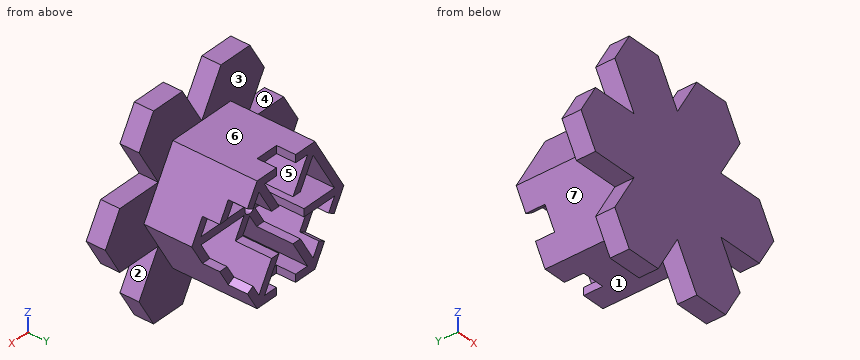
from build123d import *

# Parameters (mm, degrees)
SALIENTE_EXTRUIR1_DEPTH = 10
SALIENTE_EXTRUIR2_DEPTH = 170
CORTAR_EXTRUIR1_DEPTH   = 4
MATRIZC1_COUNT          = 5
MATRIZC1_ANGLE          = 240
CROQUIS4_W              = 24
CROQUIS4_H              = 12
SALIENTE_EXTRUIR3_DEPTH = 36
CROQUIS5_W              = 24
CROQUIS5_H              = 9
CORTAR_EXTRUIR2_DEPTH   = 24
CHAFL_N1_SIZE2          = 36
CHAFL_N1_SIZE           = 98.9091871
CORTAR_EXTRUIR3_DEPTH   = 24
CROQUIS7_W              = 30
CROQUIS7_H              = 18
CROQUIS7_R              = 3
SALIENTE_EXTRUIR4_DEPTH = 3
CROQUIS8_W              = 150
CROQUIS8_H              = 150
CORTAR_EXTRUIR4_DEPTH   = 130
CROQUIS9_W              = 64.5
CROQUIS9_H              = 23
CORTAR_EXTRUIR5_DEPTH   = 19
CROQUIS10_R             = 3
CORTAR_EXTRUIR6_DEPTH   = 8


with BuildPart() as part:
    # Croquis1 → Saliente-Extruir1 (new body)
    with BuildSketch(Plane(origin=(0, 0, 0), x_dir=(1, 0, 0), z_dir=(0, 1, 0))):
        Polygon((-12, 51.961524227), (-30, 51.961524227), (-39, 36.373066959), (-27, 15.588457268), (-51, 15.588457268), (-60, 0), (-51, -15.588457268), (-27, -15.588457268), (-39, -36.373066959), (-30, -51.961524227), (-12, -51.961524227), (0, -31.176914536), (12, -51.961524227), (30, -51.961524227), (39, -36.373066959), (27, -15.588457268), (51, -15.588457268), (60, 0), (51, 15.588457268), (27, 15.588457268), (39, 36.373066959), (30, 51.961524227), (12, 51.961524227), (0, 31.176914536), align=None)
    extrude(amount=SALIENTE_EXTRUIR1_DEPTH)

    # Croquis2 → Saliente-Extruir2 (add)
    # profile 1 of 2: a face of its own
    with BuildSketch(Plane(origin=(0, 10, 0), x_dir=(1, 0, 0), z_dir=(0, 1, 0))):
        Polygon((36, 0), (18, 31.176914536), (-18, 31.176914536), (-36, 0), (-18, -31.176914536), (18, -31.176914536), align=None)
        Polygon((15.690598923, 27.176914536), (-15.690598923, 27.176914536), (-31.381197846, 0), (-15.690598923, -27.176914536), (15.690598923, -27.176914536), (31.381197846, 0), align=None, mode=Mode.SUBTRACT)
    # profile 2 of 2: a face of its own
    with BuildSketch(Plane(origin=(0, 10, 0), x_dir=(1, 0, 0), z_dir=(0, 1, 0))):
        Polygon((-13.381197846, 27.176914536), (-15.690598923, 27.176914536), (-16.845299462, 25.176914536), (-3.464101615, 2), (-30.226497308, 2), (-31.381197846, 0), (-30.226497308, -2), (-3.464101615, -2), (-16.845299462, -25.176914536), (-15.690598923, -27.176914536), (-13.381197846, -27.176914536), (0, -4), (13.381197846, -27.176914536), (15.690598923, -27.176914536), (16.845299462, -25.176914536), (3.464101615, -2), (30.226497308, -2), (31.381197846, 0), (30.226497308, 2), (3.464101615, 2), (16.845299462, 25.176914536), (15.690598923, 27.176914536), (13.381197846, 27.176914536), (0, 4), align=None)
    extrude(amount=SALIENTE_EXTRUIR2_DEPTH)

    # Croquis3 → Cortar-Extruir1 (cut)
    with BuildSketch(Plane.XY.offset(31.176914536)):
        Polygon((-14, 172), (-2, 172), (6, 164), (6, 44), (-6, 44), (-6, 159.029437252), (-6.970562748, 160), (-14, 160), align=None)
    cortar_extruir1 = extrude(amount=-CORTAR_EXTRUIR1_DEPTH, mode=Mode.SUBTRACT)

    # MatrizC1: Cortar-Extruir1 ×5 about axis
    matrizc1_axis = Axis((0, 0, 0), (0, 1, 0))
    for i in range(1, MATRIZC1_COUNT):
        add(cortar_extruir1.rotate(matrizc1_axis, i * MATRIZC1_ANGLE / (MATRIZC1_COUNT - 1)), mode=Mode.SUBTRACT)

    # Croquis4 → Saliente-Extruir3 (add)
    with BuildSketch(Plane(origin=(-27, 0, 15.588457268), x_dir=(0.5000000000000002, 0, 0.8660254037844386), z_dir=(-0.8660254037844386, 0, 0.5000000000000002))):
        with Locations((0, 172)):
            Rectangle(CROQUIS4_W, CROQUIS4_H)
    extrude(amount=SALIENTE_EXTRUIR3_DEPTH)

    # Croquis5 → Cortar-Extruir2 (cut)
    with BuildSketch(Plane(origin=(-58.176914536, 0, 33.588457268), x_dir=(0.5000000000000003, 0, 0.8660254037844386), z_dir=(-0.8660254037844385, 0, 0.5000000000000002))):
        with Locations((0, 173.5)):
            Rectangle(CROQUIS5_W, CROQUIS5_H)
    extrude(amount=-CORTAR_EXTRUIR2_DEPTH, mode=Mode.SUBTRACT)

    # Chaflán1
    chafl_n1_edges = [part.edges().sort_by_distance(p)[0] for p in [
        (-27, 166, 15.588457268),
    ]]
    chafl_n1_side = [part.faces().sort_by_distance(p)[0] for p in [
        (-27, 165.28, 15.588457268),
    ]]
    chamfer(chafl_n1_edges, length=CHAFL_N1_SIZE - 0.0001, length2=CHAFL_N1_SIZE2 - 0.0001, reference=chafl_n1_side[0])  # a hair under: the kernel refuses the full size

    # Croquis6 → Cortar-Extruir3 (cut)
    with BuildSketch(Plane(origin=(-6, 0, -10.392304845), x_dir=(-0.8660254037844385, 0, 0.5000000000000003), z_dir=(-0.5000000000000003, 0, -0.8660254037844385))):
        Polygon((58.663492356, 166), (31.176914536, 90.481248101), (31.176914536, 166), align=None)
    extrude(amount=-CORTAR_EXTRUIR3_DEPTH, mode=Mode.SUBTRACT)

    # Croquis7 → Saliente-Extruir4 (add)
    with BuildSketch(Plane(origin=(-58.176914536, 0, 33.588457268), x_dir=(0.5000000000000003, 0, 0.8660254037844386), z_dir=(-0.8660254037844385, 0, 0.5000000000000002))):
        with Locations((-3, 175)):
            Rectangle(CROQUIS7_W, CROQUIS7_H)
        with Locations((-3, 175)):
            Circle(CROQUIS7_R, mode=Mode.SUBTRACT)
    extrude(amount=-SALIENTE_EXTRUIR4_DEPTH)

    # Croquis8 → Cortar-Extruir4 (cut)
    with BuildSketch(Plane(origin=(0, 184, 0), x_dir=(1, 0, 0), z_dir=(0, 1, 0))):
        Rectangle(CROQUIS8_W, CROQUIS8_H)
    extrude(amount=-CORTAR_EXTRUIR4_DEPTH, mode=Mode.SUBTRACT)

    # Croquis9 → Cortar-Extruir5 (cut)
    with BuildSketch(Plane(origin=(0, 54, 0), x_dir=(1, 0, 0), z_dir=(0, 1, 0))):
        with Locations((21.05, 0)):
            Rectangle(CROQUIS9_W, CROQUIS9_H)
    extrude(amount=-CORTAR_EXTRUIR5_DEPTH, mode=Mode.SUBTRACT)

    # Croquis10 → Cortar-Extruir6 (cut)
    with BuildSketch(Plane(origin=(0, 35, 0), x_dir=(1, 0, 0), z_dir=(0, 1, 0))):
        with Locations(Location((0, 0, 0), (0, 0, 270))):
            Circle(CROQUIS10_R)
    extrude(amount=-CORTAR_EXTRUIR6_DEPTH, mode=Mode.SUBTRACT)


solid = part.part
Part model, mm, in its own coordinate system. Face numbers are marked on the shaded views. A direction names the side the tool comes from. Round coordinates to 2 decimals unless told otherwise and drop trailing zeros. Loops run counter-clockwise (first coordinate to the right, second up) from the corner with the lowest first, then second, coordinate; pieces in that order, holes last. Notation, with made-up numbers: (26.5, -26) - (32.5, -26) arc R6 ccw to (32.5, -18) - close; hole circle Ø11 at (-37, 30.25). An arc over 180 degrees is marked (long way). Answer as a JSON object with one key per item and string values.
Item 1: Band-saw the part on D-D on y = 8.5. List the corners of the cut face in (x, z), plus the area to 3 significant figures.
Output:
{"outline": "(-60, 0) - (-51, -15.59) - (-27, -15.59) - (-39, -36.37) - (-30, -51.96) - (-12, -51.96) - (0, -31.18) - (12, -51.96) - (30, -51.96) - (39, -36.37) - (27, -15.59) - (51, -15.59) - (60, 0) - (51, 15.59) - (27, 15.59) - (39, 36.37) - (30, 51.96) - (12, 51.96) - (0, 31.18) - (-12, 51.96) - (-30, 51.96) - (-39, 36.37) - (-27, 15.59) - (-51, 15.59) - close", "area": "7,860 mm2"}
Item 2: Pull direction X, two halves, no side cores. Call the marked faces 5, 6 and 7: pulls with the +X half, pulls with the -X half, needs draft (parallel to the pull), parting line crosses it, or undercut.
Output:
{"face 5": "undercut", "face 6": "needs draft", "face 7": "pulls with the -X half"}
Item 3: Wall check: L1, parallel to X at y = 29, z = 0; L2, parallel to Z at x = -33.5, y = 4.5; L3, parallel to Z at x = -25.5, y = 37. Give the ranges that are in metal, low to high.
Output:
{"L1": "-36 to -3, 3 to 36", "L2": "-45.9 to -26.85, -15.59 to 15.59, 26.85 to 45.9", "L3": "-18.19 to -10.19, -2 to 2, 10.19 to 18.19"}
Item 4: Band-saw the part on A-A on z = 44.5. List the corners of the cut face in (x, y), plus the area to 3 significant figures.
Output:
{"outline": "(-34.31, 0) - (-7.69, 0) - (-7.69, 10) - (-34.31, 10) - close; (7.69, 0) - (34.31, 0) - (34.31, 10) - (7.69, 10) - close", "area": "532 mm2"}
Item 5: Pin check, flat tips, straight feed: pin 1 (13.5 mm diameter, centred on x = -20.5, y = 33.5, fed in from +Z); pin 2 (12 mm diameter, centred on y = 38, z = 28.5, fed in from -X); pin 3 (4 mm diameter, centred on y = 29.5, z = -13.5, fed in from +X). Stop position of each tip, or through.
Output:
{"pin 1": "z = 31.18", "pin 2": "x = -23.01", "pin 3": "x = 29.36"}
Item 6: Band-saw the part on C-C on y = 30. List the corners of the cut face in (x, z), plus the area to 3 significant figures.
Output:
{"outline": "(-36, 0) - (-18, -31.18) - (18, -31.18) - (36, 0) - (18, 31.18) - (-18, 31.18) - close; hole (-30.23, -2) - (-16.85, -25.18) - (-3.46, -2) - close; hole (-30.23, 2) - (-3.46, 2) - (-16.85, 25.18) - close; hole (-13.38, -27.18) - (13.38, -27.18) - (0, -4) - close; hole (-13.38, 27.18) - (0, 4) - (13.38, 27.18) - close; hole circle Ø6 at (0, 0); hole (3.46, -2) - (16.85, -25.18) - (30.23, -2) - close; hole (3.46, 2) - (30.23, 2) - (16.85, 25.18) - close", "area": "1,480 mm2"}
Item 7: Band-saw the part on B-B on x = -32. List the corners of the cut face in (y, z).
Output:
{"outline": "(0, -48.5) - (10, -48.5) - (10, -24.25) - (0, -24.25) - close; (0, -15.59) - (10, -15.59) - (10, -6.93) - (54, -6.93) - (54, 6.93) - (10, 6.93) - (10, 15.59) - (0, 15.59) - close; (0, 24.25) - (10, 24.25) - (10, 48.5) - (0, 48.5) - close"}
Item 8: Tool access for the marked faces 1, 2, 3 and 4: list every direction of +Z, -Z, +X, -X, +Y, -Y with a clear straight run to the whole face (end or side of a thin tool).
Output:
{"face 1": "-Z, +X, -X, +Y", "face 2": "+X, +Y, -Y", "face 3": "+Z, -X, +Y", "face 4": "-X, +Y, -Y"}
